Design review of the part built by this model. Coordinates are the model's own, in mm. Face numbers are marked on the shaded views. A direction names the side the tool comes from. Give positions to 0.01 mm unless a question says otherwise; leave off trailing zeros. Order: outer loops, then holes, each group sorted by start corner. A loop starts at its lowest first (then second) coordinate and runs counter-clockwise, first axis right, second up. Notation, with made-up numbers: (36, 81) - (47, 81) arc R12 ccw to (47, 100) - close; hole circle Ø2 at (-31, -12). An arc over 180 degrees is marked (long way). Write each question's results on one line, items separated by ' | '. Start each with the question number.
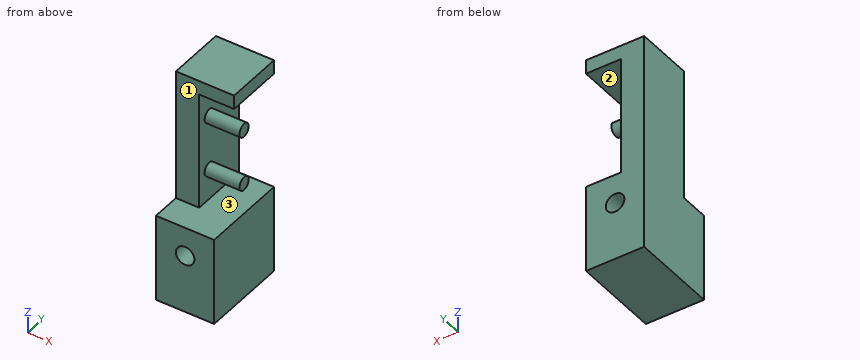
```python
from build123d import *

# Parameters (mm, degrees)
EXTRUDE_1_DEPTH     = 5
SKETCH_2_W          = 20.2
SKETCH_2_H          = 10
CUT_EXTRUDE_1_DEPTH = 6
SKETCH_3_R          = 1.15
EXTRUDE_2_DEPTH     = 6
CUT_EXTRUDE_2_REACH = 17
SKETCH_5_R          = 1.6


with BuildPart() as part:
    # 草图1 → 凸台-拉伸1 (new body, symmetric)
    with BuildSketch(Plane(origin=(0, 0, 0), x_dir=(0, 0, -1), z_dir=(1, 0, 0))):
        Polygon((0, 0), (15, 0), (15, 15), (-22.6, 15), (-22.6, 5), (0, 5), (0, 4), align=None)
    extrude(amount=EXTRUDE_1_DEPTH, both=True)

    # 草图2 → 切除-拉伸1 (cut)
    with BuildSketch(Plane(origin=(5, 0, 0), x_dir=(0, 0, -1), z_dir=(1, 0, 0))):
        with Locations((-10.1, 10)):
            Rectangle(SKETCH_2_W, SKETCH_2_H)
    extrude(amount=-CUT_EXTRUDE_1_DEPTH, mode=Mode.SUBTRACT)

    # 草图3 → 凸台-拉伸2 (add)
    with BuildSketch(Plane(origin=(-1, 0, 0), x_dir=(0, 0, -1), z_dir=(1, 0, 0))):
        with Locations((-14.85, 7.5)):
            Circle(SKETCH_3_R)
        with Locations((-5.35, 7.5)):
            Circle(SKETCH_3_R)
    extrude(amount=EXTRUDE_2_DEPTH)

    # 草图5 → 切除-拉伸2 (cut, up to next)
    with BuildSketch(Plane.XZ, mode=Mode.PRIVATE) as cut_extrude_2_sk1:
        with Locations((0, -5)):
            Circle(SKETCH_5_R)
    cut_extrude_2_tool1 = extrude(cut_extrude_2_sk1.sketch, amount=-CUT_EXTRUDE_2_REACH, mode=Mode.PRIVATE) & part.part
    add(cut_extrude_2_tool1.solids().sort_by_distance((0, 0, -5))[0], mode=Mode.SUBTRACT)


solid = part.part
```
Q1. Add section B-B (x = 2.25). Give the boundary of the cut face in (y, z).
Q2. For line 1 (Z direction, x = 0, y = 9.25); line 2 (Z direction, x = 4.75, y = 11.5); line 3 (Z direction, x = 0, y = 8.5), list the stretches that pass through material, from the lowest coordinate up. Write a range as [from, to].
Q3. Add section D-D (x = 0). Give the boundary of the cut face in (y, z), plus the area to 3 significant figures.
Q4. Machinability: for the marked faces 1, 2 and 3, which of the approach directions +Z, -Z, +X, -X, +Y, -Y give a long, thin tool a straight path to every point of the face, cutting with its end or side? Answer none if there is none.
Q5. Insertion check: pin 1 Ø4 at (y, z) = (11, 2.5) entering from +X; pin 2 Ø4 at (x, y) = (1.5, 2) entering from +Z; pin 3 Ø5 at (x, z) = (-3.5, 4) entering from -Y; pin 4 Ø4 at (y, z) = (2, 17) entering from -X. Each pin has a flat end and moves straight along its axis. Give the tip position at first contact, or say it passes through.
Q6. Add section A-A (y = 7.5). Give the boundary of the cut face in (x, z), plus the area to 3 significant figures.
Q7. Add section C-C (z = -5). Give the boundary of the cut face in (x, y), plus the area to 3 significant figures.
Verdict:
1) outline: (0, -15) - (15, -15) - (15, 0) - (0, 0) - close; (5, 20.2) - (15, 20.2) - (15, 22.6) - (5, 22.6) - close; circle Ø2.3 at (7.5, 5.35); circle Ø2.3 at (7.5, 14.85)
2) line 1: z = [-15, -6.6], [-3.4, 0], [20.2, 22.6] | line 2: z = [-15, 0], [20.2, 22.6] | line 3: z = [-15, -6.6], [-3.4, 0], [4.78, 5.92], [14.28, 15.42], [20.2, 22.6]
3) outline: (0, -15) - (15, -15) - (15, -6.6) - (0, -6.6) - close; (0, -3.4) - (15, -3.4) - (15, 0) - (0, 0) - close; (5, 20.2) - (15, 20.2) - (15, 22.6) - (5, 22.6) - close; circle Ø2.3 at (7.5, 5.35); circle Ø2.3 at (7.5, 14.85) | area: 209 mm2
4) face 1: +Z, +X, -X, -Y | face 2: +X, +Y, -Y | face 3: +X, -Y
5) pin 1: stops at x = -1 | pin 2: stops at z = 0 | pin 3: stops at y = 5 | pin 4: passes through
6) outline: (-5, -15) - (5, -15) - (5, 0) - (-1, 0) - (-1, 4.2) - (5, 4.2) - (5, 6.5) - (-1, 6.5) - (-1, 13.7) - (5, 13.7) - (5, 16) - (-1, 16) - (-1, 20.2) - (5, 20.2) - (5, 22.6) - (-5, 22.6) - close; hole circle Ø3.2 at (0, -5) | area: 274 mm2
7) outline: (-5, 0) - (-1.6, 0) - (-1.6, 15) - (-5, 15) - close; (1.6, 0) - (5, 0) - (5, 15) - (1.6, 15) - close | area: 102 mm2
